Can you work these out from the model? Positions are in its coordinate system, mm. A direction names the side the tool comes from. Give positions to 0.01 mm unless a question says otherwise; leave off trailing zeros. Order: outer loops, then holes, each group sorted by start corner. A loop starts at its lowest first (then second) coordinate and runs counter-clockwise, first axis right, second up. Notation, with made-up numbers: (18, -12.75) - (75, -12.75) arc R31 cw to (75, 26.25) - close; hole circle Ø1 at (34, 13). An arc over 180 degrees is marked (long way). One line per question, with ' | ' between items.
```python
from build123d import *

# Parameters (mm, degrees)
F0_R     = 11.2
F1_DEPTH = 7


with BuildPart() as f1:
    # F0 (on Top) → F1 (new body)
    with BuildSketch(Plane.XY):
        with BuildLine():
            Line((20.60563, 26.555137), (12.969892, 33.086074))
            ThreePointArc((12.969892, 33.086074), (13.174742, 36.356221), (12.567829, 39.576077))
            ThreePointArc((12.567829, 39.576077), (11.886143, 41.281075), (10.974449, 42.874979))
            ThreePointArc((10.974449, 42.874979), (-1.966663, 48.592701), (-12.648497, 39.315678))
            Line((-12.648497, 39.315678), (-13.099321, 37.167231))
            ThreePointArc((-13.099321, 37.167231), (-13.135205, 34.233743), (-12.522272, 31.364779))
            Line((-12.522272, 31.364779), (-21.996098, 28.017505))
            ThreePointArc((-21.996098, 28.017505), (-24.725703, 29.829983), (-27.817638, 30.914309))
            Line((-27.817638, 30.914309), (-31.47126, 31.183852))
            ThreePointArc((-31.47126, 31.183852), (-42.893509, 22.835381), (-40.200288, 8.94613))
            ThreePointArc((-40.200288, 8.94613), (-39.41319, 8.179754), (-38.565091, 7.481482))
            ThreePointArc((-38.565091, 7.481482), (-36.042557, 5.983661), (-33.251495, 5.079996))
            Line((-33.251495, 5.079996), (-35.089584, -4.798216))
            ThreePointArc((-35.089584, -4.798216), (-38.024038, -6.255884), (-40.509059, -8.391415))
            ThreePointArc((-40.509059, -8.391415), (-41.644788, -9.834271), (-42.569301, -11.420773))
            ThreePointArc((-42.569301, -11.420773), (-41.050438, -25.486966), (-27.675384, -30.099194))
            ThreePointArc((-27.675384, -30.099194), (-26.618133, -29.800735), (-25.589362, -29.415396))
            ThreePointArc((-25.589362, -29.415396), (-23.030945, -27.979728), (-20.852816, -26.01443))
            Line((-20.852816, -26.01443), (-13.217078, -32.545368))
            ThreePointArc((-13.217078, -32.545368), (-13.421928, -35.815514), (-12.815014, -39.035371))
            ThreePointArc((-12.815014, -39.035371), (-12.133329, -40.740369), (-11.221634, -42.334272))
            ThreePointArc((-11.221634, -42.334272), (1.719478, -48.051994), (12.401311, -38.774971))
            ThreePointArc((12.401311, -38.774971), (12.671463, -37.710136), (12.852135, -36.626524))
            ThreePointArc((12.852135, -36.626524), (12.888019, -33.693036), (12.275086, -30.824072))
            Line((12.275086, -30.824072), (21.748913, -27.476798))
            ThreePointArc((21.748913, -27.476798), (24.478517, -29.289276), (27.570452, -30.373602))
            ThreePointArc((27.570452, -30.373602), (29.387866, -30.635744), (31.224074, -30.643145))
            ThreePointArc((31.224074, -30.643145), (42.646323, -22.294675), (39.953102, -8.405424))
            ThreePointArc((39.953102, -8.405424), (39.166004, -7.639048), (38.317905, -6.940775))
            ThreePointArc((38.317905, -6.940775), (35.795371, -5.442955), (33.004309, -4.539289))
            Line((33.004309, -4.539289), (34.842398, 5.338923))
            ThreePointArc((34.842398, 5.338923), (37.776853, 6.796591), (40.261873, 8.932122))
            ThreePointArc((40.261873, 8.932122), (41.397602, 10.374978), (42.322116, 11.96148))
            ThreePointArc((42.322116, 11.96148), (40.803253, 26.027673), (27.428198, 30.639901))
            Line((27.428198, 30.639901), (25.342176, 29.956103))
            ThreePointArc((25.342176, 29.956103), (22.783759, 28.520435), (20.60563, 26.555137))
        make_face()
        with Locations((-0.247186, -34.999323)):
            Circle(F0_R, mode=Mode.SUBTRACT)
        with Locations((-30.729825, -17.25745)):
            Circle(F0_R, mode=Mode.SUBTRACT)
        with BuildLine():
            Line((-16.589028, -6.209999), (-20.753169, -8.614167))
            ThreePointArc((-20.753169, -8.614167), (-24.873356, -5.427752), (-29.905395, -4.083221))
            Line((-29.905395, -4.083221), (-28.209342, 5.031667))
            ThreePointArc((-28.209342, 5.031667), (-26.705532, 5.401733), (-25.255414, 5.945381))
            Line((-25.255414, 5.945381), (-16.589028, -6.209999))
        make_face(mode=Mode.SUBTRACT)
        with BuildLine():
            ThreePointArc((-2.744161, -22.037644), (-7.563771, -24.012623), (-11.244188, -27.698231))
            Line((-11.244188, -27.698231), (-18.289886, -21.671962))
            ThreePointArc((-18.289886, -21.671962), (-17.858467, -20.184591), (-17.604222, -18.656928))
            Line((-17.604222, -18.656928), (-2.744161, -17.229308))
            Line((-2.744161, -17.229308), (-2.744161, -22.037644))
        make_face(mode=Mode.SUBTRACT)
        with BuildLine():
            Line((-18.144567, -13.276083), (-10.024378, -8.58789))
            ThreePointArc((-10.024378, -8.58789), (-6.80271, -11.312079), (-2.886078, -12.880627))
            Line((-2.886078, -12.880627), (-17.677064, -15.291378))
            ThreePointArc((-17.677064, -15.291378), (-17.871273, -14.274558), (-18.144567, -13.276083))
        make_face(mode=Mode.SUBTRACT)
        with BuildLine():
            Line((2.597478, -22.109486), (2.597478, -12.941913))
            ThreePointArc((2.597478, -12.941913), (6.561509, -11.453672), (9.850395, -8.786907))
            Line((9.850395, -8.786907), (4.576526, -22.712264))
            ThreePointArc((4.576526, -22.712264), (3.598829, -22.372044), (2.597478, -22.109486))
        make_face(mode=Mode.SUBTRACT)
        with BuildLine():
            ThreePointArc((17.885416, -13.153124), (17.185992, -18.314518), (18.537614, -23.344657))
            Line((18.537614, -23.344657), (9.795863, -26.433276))
            ThreePointArc((9.795863, -26.433276), (8.723471, -25.315971), (7.5276, -24.331956))
            Line((7.5276, -24.331956), (13.721275, -10.748956))
            Line((13.721275, -10.748956), (17.885416, -13.153124))
        make_face(mode=Mode.SUBTRACT)
        Circle(F0_R, mode=Mode.SUBTRACT)
        with BuildLine():
            Line((20.618452, -8.56305), (12.60023, -3.933727))
            ThreePointArc((12.60023, -3.933727), (13.196812, 0.290111), (12.415187, 4.483651))
            Line((12.415187, 4.483651), (12.555742, 4.5648))
            Line((12.555742, 4.5648), (22.129997, -7.150533))
            ThreePointArc((22.129997, -7.150533), (21.34651, -7.827133), (20.618452, -8.56305))
        make_face(mode=Mode.SUBTRACT)
        with Locations((30.359046, -17.471519)):
            Circle(F0_R, mode=Mode.SUBTRACT)
        with Locations((-30.606232, 18.012226)):
            Circle(F0_R, mode=Mode.SUBTRACT)
        with BuildLine():
            Line((-20.865638, 9.103756), (-12.490782, 4.268531))
            ThreePointArc((-12.490782, 4.268531), (-13.198662, 0.187953), (-12.607263, -3.911126))
            Line((-12.607263, -3.911126), (-12.802928, -4.024093))
            Line((-12.802928, -4.024093), (-22.377183, 7.69124))
            ThreePointArc((-22.377183, 7.69124), (-21.593695, 8.36784), (-20.865638, 9.103756))
        make_face(mode=Mode.SUBTRACT)
        with BuildLine():
            ThreePointArc((-10.043049, 26.973982), (-8.970657, 25.856677), (-7.774785, 24.872663))
            Line((-7.774785, 24.872663), (-13.96846, 11.289662))
            Line((-13.96846, 11.289662), (-18.132602, 13.69383))
            ThreePointArc((-18.132602, 13.69383), (-17.433178, 18.855224), (-18.7848, 23.885364))
            Line((-18.7848, 23.885364), (-10.043049, 26.973982))
        make_face(mode=Mode.SUBTRACT)
        with BuildLine():
            Line((-4.823712, 23.252971), (-2.844664, 22.650193))
            ThreePointArc((-2.844664, 22.650193), (-3.846015, 22.912751), (-4.823712, 23.252971))
        make_face(mode=Mode.SUBTRACT)
        with BuildLine():
            Line((17.897381, 13.81679), (9.620439, 9.038095))
            ThreePointArc((9.620439, 9.038095), (6.368403, 11.562156), (2.496975, 12.961679))
            Line((2.496975, 12.961679), (2.496975, 13.398203))
            Line((2.496975, 13.398203), (17.429879, 15.832084))
            ThreePointArc((17.429879, 15.832084), (17.624087, 14.815264), (17.897381, 13.81679))
        make_face(mode=Mode.SUBTRACT)
        with BuildLine():
            ThreePointArc((2.496975, 22.578351), (7.316585, 24.553329), (10.997002, 28.238938))
            Line((10.997002, 28.238938), (18.0427, 22.212669))
            ThreePointArc((18.0427, 22.212669), (17.611282, 20.725298), (17.357036, 19.197635))
            Line((17.357036, 19.197635), (2.496975, 17.770015))
            Line((2.496975, 17.770015), (2.496975, 22.578351))
        make_face(mode=Mode.SUBTRACT)
        with BuildLine():
            Line((29.658209, 4.623928), (27.962156, -4.49096))
            ThreePointArc((27.962156, -4.49096), (26.458346, -4.861026), (25.008228, -5.404674))
            Line((25.008228, -5.404674), (16.341842, 6.750706))
            Line((16.341842, 6.750706), (20.505983, 9.154874))
            ThreePointArc((20.505983, 9.154874), (24.62617, 5.968458), (29.658209, 4.623928))
        make_face(mode=Mode.SUBTRACT)
        with Locations((30.482639, 17.798157)):
            Circle(F0_R, mode=Mode.SUBTRACT)
        with Locations((0, 35.54003)):
            Circle(F0_R, mode=Mode.SUBTRACT)
    extrude(amount=-F1_DEPTH)


solid = f1.part
```
(1) On a 3-axis mill with a long thin cutter (end or side, diameter ignored), from which of +Z, -Z, +X, -X, +Y, -Y can I reach the whole of each face in a straight line? I mean faces 1 (the face through (-36.08, 6, -3.45)), 2 (the face through (-2.744, -20, -3)). Say none if no direction works.
Answer below:
face 1: +Z, -Z, -X | face 2: +Z, -Z
(2) Imagine slicing it at B-B (y = 0). List the corners of the cut face in (x, z) for me.
Answer below:
outline: (-34.2, -7) - (-29.15, -7) - (-29.15, 0) - (-34.2, 0) - close; (-21.02, -7) - (-16.09, -7) - (-16.09, 0) - (-21.02, 0) - close; (-13.2, -7) - (-11.2, -7) - (-11.2, 0) - (-13.2, 0) - close; (11.2, -7) - (13.2, -7) - (13.2, 0) - (11.2, 0) - close; (16.29, -7) - (21.15, -7) - (21.15, 0) - (16.29, 0) - close; (28.8, -7) - (33.85, -7) - (33.85, 0) - (28.8, 0) - close
(3) Imagine slicing it at A-A (x = 0). List the corners of the cut face in (y, z) for me, and give its area (3 significant figures).
Answer below:
outline: (-48.2, -7) - (-46.2, -7) - (-46.2, 0) - (-48.2, 0) - close; (-23.8, -7) - (-11.2, -7) - (-11.2, 0) - (-23.8, 0) - close; (11.2, -7) - (24.34, -7) - (24.34, 0) - (11.2, 0) - close; (46.74, -7) - (48.74, -7) - (48.74, 0) - (46.74, 0) - close | area: 208 mm^2
(4) If I drill on line 1 (Y direction, x = 0, z = -1.25); line 2 (Y direction, x = 30, z = -6); line 3 (X direction, y = 27.5, z = -3.5), over which ranges is the centre line in solid material (lowest first)?
Answer below:
line 1: -48.2 to -46.2, -23.8 to -11.2, 11.2 to 24.34, 46.74 to 48.74 | line 2: -30.67 to -28.67, -6.28 to 6.61, 28.99 to 30.99 | line 3: -39.78 to -36.56, -24.65 to -7.8, 7.8 to 10.47, 11.86 to 19.5, 21.53 to 24.89, 36.08 to 39.43
(5) If we mould it in two halves opening along Y, with no side actions, what happens to faces 3 (the face through (-14.5, 25.4, -3.5)), 4 (the face through (3.613, -22.376, -3.451)), 5 (the face through (29.362, -30.634, -3.451))? For each: released by +Y, released by -Y, zero draft, split by the parting line, or undercut.
Answer below:
face 3: undercut | face 4: undercut | face 5: released by -Y
(6) Will these pins go through, and if not, where does the flat tip stop? pin 1 (3 mm diameter, centred on x = 6.5, z = -1, fed in from -Y); pin 2 (2 mm diameter, centred on x = -30.5, z = -4.5, fed in from -Y); pin 3 (2 mm diameter, centred on y = -16, z = -3.5, fed in from +X).
Answer below:
pin 1: y = -47.11 | pin 2: y = -30.46 | pin 3: x = 43.55
(7) Imagine slicing it at C-C (z = -2.5). Count the separate pieces of the cut face and the enclosed holes in it, and give its area (3 significant figures).
Answer below:
separate pieces: 1 | enclosed holes: 19 | area: 2,030 mm^2
